Model file for the job. Use its own axes, mm. A direction names the side the tool comes from. Round coordinates to 2 decimals unless told otherwise and drop trailing zeros. Write each loop counter-clockwise with the first axis right and the second up, starting at its lowest first coordinate (ties: lowest second). Pieces come first, ordered by that corner, then holes.
Autodesk Fusion 360 part; units mm, degrees
sketch "スケッチ1" plane through (0, 0, 0) normal (0, 0, 1) x (1, 0, 0)
  line L0 (239.1777, -2.4183) -> (239.1601, -97.857)
  spline S0 degree 3 poles (239.1601, -97.857) (239.1855, -99.2018) (238.1172, -100.3131) (236.7725, -100.3413) knots 0 0 0 0 1 1 1 1
  line L1 (236.7725, -100.3413) -> (2.6363, -100.3547)
  spline S1 degree 3 poles (2.6363, -100.3547) (1.2915, -100.3801) (0.1799, -99.3119) (0.152, -97.9671) knots 0 0 0 0 1 1 1 1
  line L2 (0.152, -97.9671) -> (0.152, -2.5093)
  spline S2 degree 3 poles (0.152, -2.5093) (0.1266, -1.1645) (1.1949, -0.0529) (2.5393, -0.025) knots 0 0 0 0 1 1 1 1
  line L3 (2.5393, -0.025) -> (236.6931, -0.031)
  spline S3 degree 3 poles (236.6931, -0.031) (238.0382, -0.0053) (239.1498, -1.0739) (239.1777, -2.4183) knots 0 0 0 0 1 1 1 1
  line L4 (1.676, -20.726) -> (1.676, -20.98)
  line L5 (1.676, -20.98) -> (1.676, -40.4107)
  line L6 (1.676, -40.4107) -> (26.695, -40.4107)
  line L7 (26.695, -40.4107) -> (26.695, -20.7257)
  line L8 (26.695, -20.7257) -> (2.311, -20.7257)
  line L9 (2.311, -20.7257) -> (1.676, -20.726)
  line L10 (1.676, -20.726) -> (1.676, -20.98)
  line L11 (10.312, -35.204) -> (10.312, -35.458)
  line L12 (2.692, -26.06) -> (0.025, -26.06)
  line L13 (0.025, -26.06) -> (0.025, -35.458)
  line L14 (0.025, -35.458) -> (10.312, -35.458)
  line L15 (10.312, -35.458) -> (10.312, -35.204)
  line L16 (10.312, -35.204) -> (10.312, -26.06)
  line L17 (10.312, -26.06) -> (2.692, -26.06)
  line L18 (22.123, -37.236) -> (22.123, -24.282)
  line L19 (22.123, -24.282) -> (15.646, -24.282)
  line L20 (15.646, -24.282) -> (15.646, -37.236)
  line L21 (15.646, -37.236) -> (22.123, -37.236)
  circle A0 centre (155.346, -2.311) radius 1.1
  circle A1 centre (236.2447, -3.073) radius 1.1
  circle A2 centre (183.921, -97.561) radius 1.1
  circle A3 centre (2.946, -97.561) radius 1.1
  circle A4 centre (2.946, -59.461) radius 1.1
  circle A5 centre (88.798, -40.411) radius 1.1
  circle A6 centre (64.922, -97.561) radius 1.1
  circle A7 centre (160.172, -40.411) radius 1.1
  circle A8 centre (79.273, -2.565) radius 1.1
  circle A9 centre (236.372, -59.461) radius 1.1
  circle A10 centre (236.2447, -97.561) radius 1.1
  circle A11 centre (2.946, -2.819) radius 1.1
  point P0 (156.446, -2.311)
  point P1 (237.3447, -3.073)
  point P2 (185.021, -97.561)
  point P3 (4.046, -97.561)
  point P4 (4.046, -59.461)
  point P5 (89.898, -40.411)
  point P6 (66.022, -97.561)
  point P7 (161.272, -40.411)
  point P8 (80.373, -2.565)
  point P9 (237.472, -59.461)
  point P10 (237.3447, -97.561)
  point P11 (4.046, -2.819)
extrude "押し出し1" add sketch "スケッチ1" against normal blind 40 contours L0 S0 L1 S1 L2 S2 L3 S3 L4 L5 L6 L7 L8 L9 L10 L12 L14 | L2 L5 L12 L14 | L5 L11 L12 L14 L15 L16 L17 | L4 L5 L6 L7 L8 L9 L10 L11 L12 L14 L15 L16 L17 | L18 L19 L20 L21
extrude "押し出し2" cut sketch "スケッチ1" against normal blind 6 contours L2 L5 L12 L14 | L5 L11 L12 L14 L15 L16 L17
extrude "押し出し3" cut sketch "スケッチ1" against normal blind 4 contours L4 L5 L6 L7 L8 L9 L10 L11 L12 L14 L15 L16 L17
extrude "押し出し4" cut sketch "スケッチ1" against normal blind 40 contours L18 L19 L20 L21
sketch "スケッチ2" plane through (0, 0, 0) normal (1, 0, 0) x (0, 1, 0)
  line L0 (-100.355, 0) -> (-100.355, -2)
  line L1 (-100.355, -2) -> (3, -13)
  line L2 (-7.5019, -11.8823) -> (0.5, -9)
  line L3 (-100.355, -2) -> (-100.57, -2)
  line L4 (-100.57, -2) -> (-100.57, -3.4)
  line L5 (-100.57, -3.4) -> (-100.57, -40.4093)
  line L6 (-100.57, -40.4093) -> (-74, -40.4093)
  line L7 (-74, -40.4093) -> (1, -40.4093)
  line L8 (1, -40.4093) -> (0.5, -9)
  dimension "d9" = 2
extrude "押し出し5" cut sketch "スケッチ2" along normal blind 400 contours L1 L3 L4 L5 L6 L7 L8
extrude "押し出し6" cut sketch "スケッチ2" along normal blind 400 contours L1 L2 L8
sketch "スケッチ3" plane through (0, 0, 0) normal (1, 0, 0) x (0, 1, 0)
  line L0 (0.1398, 0.1029) -> (-26.06, 0.1029)
sketch "スケッチ4" plane through (0, -1.3345, -12.5387) normal (0, -0.1058, -0.9944) x (1, 0, 0)
  ellipse E0 centre (160.172, 39.2973) end of major axis (160.172, 38.1911) minor radius 1.1
  ellipse E1 centre (236.2447, 96.77) end of major axis (236.2447, 95.6638) minor radius 1.1
  ellipse E2 centre (183.921, 96.77) end of major axis (183.921, 95.6638) minor radius 1.1
  ellipse E3 centre (236.372, 58.4548) end of major axis (236.372, 57.3487) minor radius 1.1
  ellipse E4 centre (88.798, 39.2973) end of major axis (88.798, 38.1911) minor radius 1.1
  ellipse E5 centre (2.946, 96.77) end of major axis (2.946, 95.6638) minor radius 1.1
  ellipse E6 centre (2.946, 58.4548) end of major axis (2.946, 57.3487) minor radius 1.1
  ellipse E7 centre (64.922, 96.77) end of major axis (64.922, 95.6638) minor radius 1.1
  line L0 (22.123, 36.1043) -> (22.123, 23.0772)
  line L1 (22.123, 23.0772) -> (15.646, 23.0772)
  line L2 (15.646, 23.0772) -> (15.646, 36.1043)
  line L3 (15.646, 36.1043) -> (22.123, 36.1043)
  line L4 (0.152, 6.2022) -> (239.1768, 6.2022)
  line L5 (239.1768, 6.2022) -> (239.1601, 97.0677)
  spline S0 degree 3 poles (236.7725, 99.566) (236.9396, 99.5624) (237.1056, 99.542) (237.4266, 99.4681) (237.5804, 99.4159) (238.0207, 99.2151) (238.2841, 99.0244) (238.7171, 98.5588) (238.8855, 98.2893) (239.1117, 97.6993) (239.166, 97.3855) (239.1601, 97.0677) knots -0.385662 -0.385662 -0.385662 -0.385662 -0.335417 -0.335417 -0.286659 -0.286659 -0.189937 -0.189937 -0.095378 -0.095378 0 0 0 0
  line L6 (236.7725, 99.566) -> (2.6363, 99.5794)
  spline S1 degree 3 poles (2.6151, 99.5798) (2.6222, 99.5797) (2.6292, 99.5796) (2.6363, 99.5794) knots -0.002119 -0.002119 -0.002119 -0.002119 0 0 0 0
  line L7 (2.6151, 99.5798) -> (2.5636, 99.5798)
  spline S2 degree 3 poles (0.152, 97.1784) (0.1556, 97.3498) (0.1766, 97.52) (0.2528, 97.8488) (0.3067, 98.0062) (0.5108, 98.4494) (0.702, 98.7126) (1.1661, 99.1426) (1.4326, 99.3091) (1.9922, 99.5233) (2.2757, 99.5767) (2.5636, 99.5798) knots -0.385525 -0.385525 -0.385525 -0.385525 -0.334027 -0.334027 -0.284114 -0.284114 -0.187392 -0.187392 -0.093864 -0.093864 -0.00728 -0.00728 -0.00728 -0.00728
  line L8 (0.152, 97.1784) -> (0.152, 6.2022)
  circle A0 centre (2.946, 96.77) radius 2.3941
  circle A1 centre (2.946, 58.4548) radius 2.3046
  circle A2 centre (64.922, 96.77) radius 2.3483
  circle A3 centre (183.921, 96.77) radius 2.2833
  circle A4 centre (236.2447, 96.77) radius 2.2651
  circle A5 centre (236.372, 58.4548) radius 2.3236
  circle A6 centre (160.172, 39.2973) radius 2.3586
  circle A7 centre (88.798, 39.2973) radius 2.4454
extrude "押し出し7" cut sketch "スケッチ4" against normal blind 1 contours E5 | A0
extrude "押し出し8" cut sketch "スケッチ4" against normal blind 1 contours E7 | A2
extrude "押し出し9" cut sketch "スケッチ4" against normal blind 1 contours E2 | A3
extrude "押し出し10" cut sketch "スケッチ4" against normal blind 1 contours E1 | A4
extrude "押し出し11" cut sketch "スケッチ4" against normal blind 1.5 contours E6 | A1
extrude "押し出し12" cut sketch "スケッチ4" against normal blind 1.5 contours E4 | A7
extrude "押し出し13" cut sketch "スケッチ4" against normal blind 1.5 contours E0 | A6
extrude "押し出し14" cut sketch "スケッチ4" against normal blind 1.5 contours E3 | A5
sketch "スケッチ5" plane through (0, 2.9269, -8.1258) normal (0, 0.3389, -0.9408) x (-1, 0, 0)
  line L0 (-0.152, -11.0847) -> (-0.152, -5.7781)
  spline S0 degree 3 poles (-2.5393, -3.1376) (-2.3792, -3.1412) (-2.2204, -3.1611) (-1.9125, -3.2329) (-1.7647, -3.2837) (-1.3412, -3.4784) (-1.0881, -3.6623) (-0.6398, -4.1342) (-0.4566, -4.4267) (-0.2063, -5.0743) (-0.1458, -5.4243) (-0.152, -5.7781) knots -0.397498 -0.397498 -0.397498 -0.397498 -0.349267 -0.349267 -0.302241 -0.302241 -0.208829 -0.208829 -0.106159 -0.106159 0 0 0 0
  line L1 (-2.5393, -3.1376) -> (-236.6931, -3.144)
  spline S1 degree 3 poles (-239.1777, -5.6814) (-239.1738, -5.4825) (-239.1489, -5.285) (-239.0577, -4.9055) (-238.9933, -4.7246) (-238.7664, -4.2552) (-238.5683, -3.9872) (-238.1011, -3.5623) (-237.8426, -3.4012) (-237.2827, -3.1885) (-236.9901, -3.138) (-236.6931, -3.144) knots -0.395915 -0.395915 -0.395915 -0.395915 -0.3363 -0.3363 -0.278857 -0.278857 -0.179915 -0.179915 -0.08914 -0.08914 0 0 0 0
  line L2 (-239.1777, -5.6814) -> (-239.1768, -11.0847)
  line L3 (-239.1768, -11.0847) -> (-0.152, -11.0847)
  ellipse E0 centre (-155.346, -5.5674) end of major axis (-155.346, -4.3983) minor radius 1.1
  ellipse E1 centre (-2.946, -6.1074) end of major axis (-2.946, -4.9382) minor radius 1.1
  ellipse E2 centre (-236.2447, -6.3773) end of major axis (-236.2447, -5.2082) minor radius 1.1
  ellipse E3 centre (-79.273, -5.8374) end of major axis (-79.273, -4.6682) minor radius 1.1
  circle A0 centre (-2.946, -6.1074) radius 2.2782
  circle A1 centre (-79.273, -5.8374) radius 2.3234
  circle A2 centre (-155.346, -5.5674) radius 2.2538
  circle A3 centre (-236.2447, -6.3773) radius 2.2901
extrude "押し出し15" cut sketch "スケッチ5" against normal blind 1.5 contours E1 | A0
extrude "押し出し16" cut sketch "スケッチ5" against normal blind 1.5 contours E3 | A1
extrude "押し出し17" cut sketch "スケッチ5" against normal blind 1.5 contours E0 | A2
extrude "押し出し18" cut sketch "スケッチ5" against normal blind 1.5 contours E2 | A3
1) Which spindle directions (+Z, -Z, +X, -X, +Y, -Y) get a long thin tool onto all of the face, cutting with end or side? Do faces 1 (the face through (117.99, -54.58, -6.87)), 2 (the face through (1.676, -23, -2)), 3 (the face through (19, -37.236, -6)), 4 (the face through (4.2, -26.06, -4.3)), 5 (the face through (2.978, -4.25, -9.117)). Say none if no direction does.
2) Cut at B-B on y = -53.5. List the corners of the cut face in (x, z), and give its area (3 significant figures).
3) Wall check: probe 1 along Y at (x, z) = (25.5, -1); probe 2 along Z at (x, y) = (141, -18); probe 3 along Z at (x, y) = (171.5, -36). Give the ranges that are in metal, low to high.
4) Cut at C-C on x = 178. List the corners of the cut face in (y, z), and give its area (3 significant figures).
5) Pull direction X, two halves, no side cores. Call faces 6 (the face through (14, -30, -4)), 7 (the face through (5, -31, -6)): released by +X, released by -X, zero draft, split by the parting line, or undercut.
6) Flat gauge pins, fed straight in: pin 1 Ø1.5 at (y, z) = (-24.5, -4) entering from +X; pin 2 Ø2 at (x, z) = (68.5, -0.5) entering from -Y; pin 3 Ø3 at (x, y) = (85, -88.5) entering from +Z; pin 4 Ø4.5 at (x, z) = (116.5, -6.5) entering from +Y. Where does each tip first touch, or does it go through?
7) Cut at A-A on x = 69.5. List the corners of the cut face in (y, z), and give its area (3 significant figures).
8) Cut at D-D on y = -82.5. List the corners of the cut face in (x, z), and give its area (3 significant figures).
Result sheet:
1. face 1: -Z, +X, -X, -Y
1. face 2: +Z
1. face 3: +Z, -Z
1. face 4: +Z, -X
1. face 5: none
2. outline: (0.15, -6.99) - (239.17, -6.99) - (239.17, 0) - (0.15, 0) - close
2. area: 1,670 mm2
3. probe 1: y = -100.35 to -40.41, -20.73 to -0.03
3. probe 2: z = -10.76 to 0
3. probe 3: z = -8.85 to 0
4. outline: (-100.34, -2) - (-7.5, -11.88) - (-0.03, -9.19) - (-0.03, 0) - (-100.34, 0) - close
4. area: 723 mm2
5. face 6: undercut
5. face 7: zero draft
6. pin 1: stops at x = 239.17
6. pin 2: stops at y = -100.35
6. pin 3: stops at z = 0
6. pin 4: stops at y = -0.03
7. outline: (-100.35, -2) - (-7.5, -11.88) - (-0.03, -9.19) - (-0.03, 0) - (-100.35, 0) - close
7. area: 723 mm2
8. outline: (0.15, -3.9) - (239.16, -3.9) - (239.16, 0) - (0.15, 0) - close
8. area: 932 mm2
